Design review of the part built by this model. Coordinates are the model's own, in mm. A direction names the side the tool comes from. Round coordinates to 2 decimals unless told otherwise and drop trailing zeros. Loops run counter-clockwise (first coordinate to the right, second up) from the corner with the lowest first, then second, coordinate; pieces in that order, holes last. Notation, with made-up numbers: (85, -39) -> (143, -39) arc R32 ccw to (143, 0) -> close; hole circle Ø8 at (73.5, -12.5). An arc over 180 degrees is marked (long way). Answer as CSV lines item,"result". Start each with the question number.
```python
from build123d import *

# Parameters (mm, degrees)
BOSS_EXTRUDE1_DEPTH = 28
BOSS_EXTRUDE2_DEPTH = 28
SKETCH5_W           = 20.4
SKETCH5_H           = 20.4
CUT_EXTRUDE3_DEPTH  = 30
CUT_EXTRUDE4_DEPTH  = 20.4
SKETCH7_R           = 2.6
CUT_EXTRUDE5_DEPTH  = 57.903989341
SKETCH8_W           = 20
SKETCH8_H           = 20
CUT_EXTRUDE6_DEPTH  = 60.150040009
SKETCH9_W           = 4
SKETCH9_H           = 20
BOSS_EXTRUDE3_DEPTH = 20
BOSS_EXTRUDE4_DEPTH = 15
SKETCH11_R          = 2.6
CUT_EXTRUDE7_DEPTH  = 65.43228341
SKETCH12_R          = 6
CUT_EXTRUDE8_DEPTH  = 62.836477907
FILLET1_R           = 3
FILLET2_R           = 6


with BuildPart() as part:
    # Sketch1 → Boss-Extrude1 (new body)
    with BuildSketch(Plane(origin=(0, 0, 0), x_dir=(0, 0, -1), z_dir=(1, 0, 0))):
        Polygon((0, 0), (-24, 0), (-24, -4), (-4, -4), (-4, -24), (0, -24), align=None)
    extrude(amount=BOSS_EXTRUDE1_DEPTH)

    # Sketch2 → Boss-Extrude2 (add)
    with BuildSketch(Plane(origin=(28, 0, 0), x_dir=(0, 0, -1), z_dir=(1, 0, 0))):
        Polygon((2.309401077, -24), (30.582903769, 24.97114317), (6.334192463, 38.97114317), (-16.165807537, 0), (0, 0), (0, -24), align=None)
    extrude(amount=-BOSS_EXTRUDE2_DEPTH)

    # Sketch5 → Cut-Extrude3 (cut)
    with BuildSketch(Plane(origin=(0, 31.97114317, -18.458548116), x_dir=(1, 0, 0), z_dir=(0, 0.8660254037844402, -0.4999999999999977))):
        with Locations((14, 0)):
            Rectangle(SKETCH5_W, SKETCH5_H)
    extrude(amount=-CUT_EXTRUDE3_DEPTH, mode=Mode.SUBTRACT)

    # Sketch6 → Cut-Extrude4 (cut)
    with BuildSketch(Plane(origin=(3.8, 0, 0), x_dir=(0, 0, -1), z_dir=(1, 0, 0))):
        Polygon((12.292007234, 0.890381057), (3.458548116, 5.990381057), (3.458548116, -14.409618943), align=None)
    extrude(amount=CUT_EXTRUDE4_DEPTH, mode=Mode.SUBTRACT)

    # Sketch7 → Cut-Extrude5 (cut, through all)
    with BuildSketch(Plane(origin=(28, 0, 0), x_dir=(0, 0, -1), z_dir=(1, 0, 0))):
        with Locations((8.458548116, 14.650635095)):
            Circle(SKETCH7_R)
    extrude(amount=-CUT_EXTRUDE5_DEPTH, mode=Mode.SUBTRACT)

    # Sketch8 → Cut-Extrude6 (cut, through all)
    with BuildSketch(Plane.XY.offset(4)):
        with Locations((14, -14)):
            Rectangle(SKETCH8_W, SKETCH8_H)
    extrude(amount=-CUT_EXTRUDE6_DEPTH, mode=Mode.SUBTRACT)

    # Sketch9 → Boss-Extrude3 (add)
    with BuildSketch(Plane.XY.offset(4)):
        with Locations((2, -14)):
            Rectangle(SKETCH9_W, SKETCH9_H)
        with Locations((26, -14)):
            Rectangle(SKETCH9_W, SKETCH9_H)
    extrude(amount=BOSS_EXTRUDE3_DEPTH)

    # Sketch10 → Boss-Extrude4 (add)
    with BuildSketch(Plane.XY.offset(24)):
        Polygon((0, 0), (28, 0), (28, -24), (24, -24), (24, -4), (4, -4), (4, -24), (0, -24), align=None)
    extrude(amount=BOSS_EXTRUDE4_DEPTH)

    # Sketch11 → Cut-Extrude7 (cut, through all)
    with BuildSketch(Plane.XZ.offset(4)):
        with Locations(Location((14, 29, 0), (0, 0, 270))):
            Circle(SKETCH11_R)
        with Locations(Location((14, 14, 0), (0, 0, 270))):
            Circle(SKETCH11_R)
    extrude(amount=-CUT_EXTRUDE7_DEPTH, mode=Mode.SUBTRACT)

    # Sketch12 → Cut-Extrude8 (cut, through all)
    with BuildSketch(Plane(origin=(0, 0, 0), x_dir=(1, 0, 0), z_dir=(0, 1, 0))):
        with Locations((14, -14)):
            Circle(SKETCH12_R)
    extrude(amount=CUT_EXTRUDE8_DEPTH, mode=Mode.SUBTRACT)

    # Fillet1
    fillet1_edges = [part.edges().sort_by_distance(p)[0] for p in [
        (23.797734696, 0, 16.165807537),
        (4.202265304, 0, 16.165807537),
    ]]
    fillet(fillet1_edges, radius=FILLET1_R)

    # Fillet2
    fillet2_edges = [part.edges().sort_by_distance(p)[0] for p in [
        (2, -24, -2.309401077),
        (26, -24, -2.309401077),
    ]]
    fillet(fillet2_edges, radius=FILLET2_R)


solid = part.part
```
Q1. Add section C-C, the plane y = -16. Give the boundary of the cut face in (x, z).
Q2. For pin 1 Ø3 at (y, z) = (14.65, -8.46) entering from +X; pin 2 Ø8 at (x, z) = (7.5, -14) entering from +Y; pin 3 Ø14 at (x, z) = (12, 27.5) entering from +Y; pin 4 Ø16.5 at (x, y) = (13.5, -5) entering from -Z, all flat-tipped, find the tip position at first contact; note any pin that passes through.
Q3. Add section A-A, the plane z = 29. Give the boundary of the cut face in (x, y).
Q4. Add section B-B, the plane x = 14. Give the boundary of the cut face in (y, z), and give its area (3 significant figures).
Q5. To check wall thickness, follow probe 1 along X at (y, z) = (-2.25, 29); probe 2 along Y at (x, z) = (16.25, 22); probe 3 along Z at (x, y) = (8.5, 0.5). State the ranges of each line that lie inside material, in increasing order. Write a range as from..to.
Q6. Machinability: for faces 1 (the flat face through (13.857, 8.505, 0.896)), 2 (the cylindrical face through (23.2, 0.4, 16.4)), 3 (the flat face through (4, -14, 18)), which of the approach directions +Z, -Z, +X, -X, +Y, -Y give a long, thin tool a straight path to every point of the face, cutting with its end or side? Answer none if there is none.
Q7. Add section D-D, the plane y = 10. Give the boundary of the cut face in (x, z).
Q8. Mouldability with a two-part tool opening along Z and no side actions: class faces 4 (the flat face through (3.8, 15.1, -11.2)), 5 (the cylindrical face through (4.7, 0.4, 16.4)), 6 (the flat face through (2, -24, 20)) as pulls with the +Z half, pulls with the -Z half, needs draft (parallel to the pull), parting line crosses it, or undercut.
Worked answers:
1,outline,"(0, -6.93) -> (4, -6.93) -> (4, 39) -> (0, 39) -> close; (24, -6.93) -> (28, -6.93) -> (28, 39) -> (24, 39) -> close"
2,pin 1,"passes through"
2,pin 2,"stops at y = 35.42"
2,pin 3,"stops at y = 0"
2,pin 4,"stops at z = -18.04"
3,outline,"(0, -24) -> (4, -24) -> (4, -4) -> (11.4, -4) -> (11.4, 0) -> (0, 0) -> close; (16.6, -4) -> (24, -4) -> (24, -24) -> (28, -24) -> (28, 0) -> (16.6, 0) -> close"
4,outline,"(-4, -13.86) -> (24.97, -30.58) -> (26.87, -27.29) -> (-4, -9.47) -> close; (-4, -3.46) -> (5.99, -3.46) -> (11.09, 5.37) -> (37.07, -9.63) -> (38.97, -6.33) -> (14.14, 8) -> (0, 8) -> (0, 11.4) -> (-4, 11.4) -> close; (-4, 16.6) -> (0, 16.6) -> (0, 26.4) -> (-4, 26.4) -> close; (-4, 31.6) -> (0, 31.6) -> (0, 39) -> (-4, 39) -> close"
4,area,"480 mm^2"
5,probe 1,"x = 0..11.4, 16.6..28"
5,probe 2,"y = -4..0"
5,probe 3,"z = -16.45..-12.07, -3.46..11.6"
6,face 1,"none"
6,face 2,"+Z, +X, -X, +Y"
6,face 3,"+Z, -Z, -Y"
7,outline,"(0, -21.94) -> (28, -21.94) -> (28, 10.39) -> (18.79, 10.39) arc R6 cw to (9.21, 10.39) -> (0, 10.39) -> close; hole (3.8, -17.55) -> (24.2, -17.55) -> (24.2, 3.49) -> (3.8, 3.49) -> close"
8,face 4,"undercut"
8,face 5,"pulls with the +Z half"
8,face 6,"needs draft"
